from build123d import *

# Parameters (mm, degrees)
EXTRUDE_1_DEPTH     = 20
SKETCH_3_W          = 210
SKETCH_3_H          = 10
CUT_EXTRUDE_1_DEPTH = 15
SKETCH_4_W          = 160
SKETCH_4_H          = 5
CUT_EXTRUDE_2_DEPTH = 10
SKETCH_5_R          = 2.5
SKETCH_5_R_2        = 2
CUT_EXTRUDE_3_DEPTH = 10
CUT_EXTRUDE_4_DEPTH = 4.3
SKETCH_8_R          = 5.75
CUT_EXTRUDE_6_DEPTH = 15
CUT_EXTRUDE_7_DEPTH = 250.048188108
CUT_EXTRUDE_START   = -8
CUT_EXTRUDE_8_DEPTH = 8


with BuildPart() as part:
    # 草图1 → 凸台-拉伸1 (new body)
    with BuildSketch(Plane.XY):
        Polygon((-115, 220), (115, 220), (60, -50), (59.592592593, -52), (-59.592592593, -52), (-60, -50), align=None)
    extrude(amount=EXTRUDE_1_DEPTH)

    # 草图3 → 切除-拉伸1 (cut)
    with BuildSketch(Plane(origin=(0, 220, 0), x_dir=(1, 0, 0), z_dir=(0, 1, 0))):
        with Locations((0, -10)):
            Rectangle(SKETCH_3_W, SKETCH_3_H)
    extrude(amount=-CUT_EXTRUDE_1_DEPTH, mode=Mode.SUBTRACT)

    # 草图4 → 切除-拉伸2 (cut)
    with BuildSketch(Plane.XY.offset(20)):
        with Locations((0, 123.51)):
            Rectangle(SKETCH_4_W, SKETCH_4_H)
    extrude(amount=-CUT_EXTRUDE_2_DEPTH, mode=Mode.SUBTRACT)

    # 草图5 → 切除-拉伸3 (cut)
    with BuildSketch(Plane.XY.offset(20)):
        with Locations((-77.25, 208.1425573)):
            Circle(SKETCH_5_R)
        with Locations((-90, 189)):
            Circle(SKETCH_5_R)
        with Locations((-64.5, 189)):
            Circle(SKETCH_5_R)
        with Locations((-55, 106.6525573)):
            Circle(SKETCH_5_R_2)
        with Locations((-67.75, 87.51)):
            Circle(SKETCH_5_R_2)
        with Locations((-42.25, 87.51)):
            Circle(SKETCH_5_R_2)
        with Locations(Location((42.25, 87.51, 0), (0, 0, 180))):
            Circle(SKETCH_5_R_2)
        with Locations(Location((67.75, 87.51, 0), (0, 0, 180))):
            Circle(SKETCH_5_R_2)
        with Locations(Location((55, 106.6525573, 0), (0, 0, 180))):
            Circle(SKETCH_5_R_2)
        with Locations(Location((64.5, 189, 0), (0, 0, 180))):
            Circle(SKETCH_5_R)
        with Locations(Location((90, 189, 0), (0, 0, 180))):
            Circle(SKETCH_5_R)
        with Locations((77.25, 208.1425573)):
            Circle(SKETCH_5_R)
    extrude(amount=-CUT_EXTRUDE_3_DEPTH, mode=Mode.SUBTRACT)

    # 草图6 → 切除-拉伸4 (cut, symmetric)
    with BuildSketch(Plane(origin=(0, 0, 10), x_dir=(-1, 0, 0), z_dir=(0, 0, -1))):
        with BuildLine():
            Line((0, -49.69), (17.486671343, -49.69))
            Line((17.486671343, -49.69), (12.108893566, -23.29))
            Line((12.108893566, -23.29), (0, -23.29))
            ThreePointArc((0, -23.29), (-13.2, -36.49), (0, -49.69))
        make_face()
    extrude(amount=CUT_EXTRUDE_4_DEPTH, both=True, mode=Mode.SUBTRACT)

    # 草图8 → 切除-拉伸6 (cut)
    with BuildSketch(Plane.XY.offset(20)):
        with Locations((0, -36.49)):
            Circle(SKETCH_8_R)
    extrude(amount=-CUT_EXTRUDE_6_DEPTH, mode=Mode.SUBTRACT)

    # 草图9 → 切除-拉伸7 (cut, through all)
    with BuildSketch(Plane.XY.offset(20)):
        with BuildLine():
            Line((13, 11.26), (47, 11.26))
            ThreePointArc((47, 11.26), (49.25, 13.51), (47, 15.76))
            Line((47, 15.76), (13, 15.76))
            ThreePointArc((13, 15.76), (10.75, 13.51), (13, 11.26))
        make_face()
    extrude(amount=-CUT_EXTRUDE_7_DEPTH, mode=Mode.SUBTRACT)

    # 草图10 → 切除-拉伸8 (cut)
    with BuildSketch(Plane(origin=(0, 0, 0), x_dir=(-1, 0, 0), z_dir=(0, 0, -1)).offset(CUT_EXTRUDE_START)):
        with BuildLine():
            Line((-50, 9.51), (-10, 9.51))
            ThreePointArc((-10, 9.51), (-6, 13.51), (-10, 17.51))
            Line((-10, 17.51), (-50, 17.51))
            ThreePointArc((-50, 17.51), (-54, 13.51), (-50, 9.51))
        make_face()
        with BuildLine():
            Line((-47, 15.76), (-13, 15.76))
            ThreePointArc((-13, 15.76), (-10.75, 13.51), (-13, 11.26))
            Line((-13, 11.26), (-47, 11.26))
            ThreePointArc((-47, 11.26), (-49.25, 13.51), (-47, 15.76))
        make_face(mode=Mode.SUBTRACT)
    extrude(amount=CUT_EXTRUDE_8_DEPTH, mode=Mode.SUBTRACT)


solid = part.part
For this review, take the finished solid that the model builds, in its own axes (mm). A direction names the side the tool comes from. Coordinates: 2 decimals unless noted, no trailing zeros. Write each loop counter-clockwise with the first axis right and the second up, starting at its lowest first coordinate (ties: lowest second). Pieces come first, ordered by that corner, then holes. Notation, with made-up numbers: (63.25, -3.5) -> (121.25, -3.5) arc R15 cw to (121.25, 0.5) -> close; hole circle Ø3 at (20, -3). An arc over 180 degrees is marked (long way). Write each question's results on one line, items separated by ' | '. Start each with the question number.
1) Consider section D-D (y = -7.5). Write out the cut boundary in (x, z).
2) Consider section C-C (y = 141.5). Write out the cut boundary in (x, z).
3) Wall thickness on L1, parallel to Y at x = 42, z = 17.5; L2, parallel to Y at x = 55, z = 16; L3, parallel to Y at x = 16.5, z = 11.25: over which ranges is each line inside the solid? List them lowest first. Write a range as [from, to].
4) For faces 1 (the face through (-9, -49.69, 10)), 2 (the face through (30, 11, 8)), 3 (the face through (-1, 205, 10)), list the 3-axis set-ups (+Z, -Z, +X, -X, +Y, -Y) from which the entire face can be reached by the end or side of a thin tool; tool diameter is ignored.
5) Consider section B-B (x = 101). Write out the cut boundary in (y, z).
6) The part is to be moulded in two halves that separate along X. For faces 4 (the face through (2, 86, 0)), 5 (the face through (-5.3, -39.2, 5.7)), say which applies: +X half, -X half, draft (parallel to the pull), parting line (faces both ways), or undercut.
7) Consider section A-A (x = 31.5). Write out the cut boundary in (y, z), plus the area to 3 significant figures.
8) Insertion check: pin 1 (1.5 mm diameter, centred on x = 63.5, y = 190, fed in from +Z); pin 2 (11 mm diameter, centred on y = 209, z = 12, fed in from -X); pin 3 (5.5 mm diameter, centred on y = 123.5, z = 17.5, fed in from -X). Each pin has a flat end and moves straight along its axis. Give the tip position at first contact, or say it passes through.
Geometry says:
1) outline: (-68.66, 0) -> (68.66, 0) -> (68.66, 20) -> (-68.66, 20) -> close
2) outline: (-99.01, 0) -> (99.01, 0) -> (99.01, 20) -> (-99.01, 20) -> close
3) L1: [-52, 11.26], [15.76, 85.53], [89.49, 121.01], [126.01, 220] | L2: [-52, 104.65], [108.65, 121.01], [126.01, 220] | L3: [-52, 11.26], [15.76, 121.01], [126.01, 205]
4) face 1: none | face 2: -Z | face 3: +Y
5) outline: (151.27, 0) -> (220, 0) -> (220, 5) -> (205, 5) -> (205, 15) -> (220, 15) -> (220, 20) -> (151.27, 20) -> close
6) face 4: draft | face 5: undercut
7) outline: (-52, 0) -> (9.51, 0) -> (9.51, 8) -> (11.26, 8) -> (11.26, 20) -> (-52, 20) -> close; (15.76, 8) -> (17.51, 8) -> (17.51, 0) -> (220, 0) -> (220, 5) -> (205, 5) -> (205, 15) -> (220, 15) -> (220, 20) -> (126.01, 20) -> (126.01, 10) -> (121.01, 10) -> (121.01, 20) -> (15.76, 20) -> close | area: 5,120 mm^2
8) pin 1: z = 10 | pin 2: x = -113.88 | pin 3: x = -95.9
